Work out the finished part from the listing and answer in its coordinate system (mm). Face numbers are marked on the shaded views. Give positions to 0.01 mm unless a question says otherwise; leave off trailing zeros. Write each loop counter-clockwise with the first axis right and the second up, starting at its lowest first coordinate (ties: lowest second). Pieces come first, ordered by that corner, then holes. Notation, with made-up numbers: (7, -32) -> (25, -32) arc R25 cw to (25, -10) -> close; hole circle Ø8 at (-21.75, 58). An arc over 180 degrees is marked (long way). Use a Markdown table: item, result. Add a question column.
Q1. For a pull along X with two mould halves and no side action, classify the marked faces 1 and 2 as pulls with the +X half, pulls with the -X half, needs draft (parallel to the pull), parting line crosses it, or undercut.
Q2. Section B-B, the plane x = -1 is taken. Give the vertices of the cut face in (y, z) (3 decimals), plus the area to 3 significant figures.
Q3. Section D-D, the plane z = 0.85 is taken. Give the vertices of the cut face in (x, y), plus the area to 3 significant figures.
Q4. Section A-A, the plane y = -2.15 is taken. Give the vertices of the cut face in (x, z) (3 decimals), plus the area to 3 significant figures.
Q5. Consider line 1 (X direction, y = 2.35, z = 0.1) (3 decimals); line 2 (Z direction, x = 2.75, y = 0); line 3 (Y direction, x = 2.25, z = 0.15). Determine where each line is inside the solid, lowest interval first.
Q6. Section C-C, the plane z = 0.4 is taken. Give the vertices of the cut face in (x, y).
from build123d import *

# Parameters (mm, degrees)
SKETCH001_W     = 5.89
SKETCH001_H     = 4.9
PAD001_DEPTH    = 1.04
POCKET_DEPTH    = 6
POCKET001_DEPTH = 6
SKETCH_W        = 0.61
SKETCH_H        = 0.41
PAD_DEPTH       = 0.05
CHAMFER004_SIZE = 0.2
CHAMFER005_SIZE = 0.2
CHAMFER006_SIZE = 0.2
CHAMFER007_SIZE = 0.2


with BuildPart() as pocket001:
    # Sketch001 → Pad001 (new body)
    with BuildSketch(Plane.XY.offset(0.05)):
        with Locations((3.075, 2.575)):
            Rectangle(SKETCH001_W, SKETCH001_H)
    extrude(amount=PAD001_DEPTH)

    # Sketch002 → Pocket (cut)
    with BuildSketch(Plane(origin=(0, 0.125, 0.05), x_dir=(1, 0, 0), z_dir=(0, -1, 0))):
        Polygon((0.13, 0.28), (0.13, 1.04), (0.291543, 1.04), align=None)
        Polygon((5.858457, 1.04), (6.02, 1.04), (6.02, 0.28), align=None)
    extrude(amount=-POCKET_DEPTH, mode=Mode.SUBTRACT)

    # Sketch003 → Pocket001 (cut)
    with BuildSketch(Plane(origin=(6.02, 0, 0.05), x_dir=(0, 1, 0), z_dir=(1, 0, 0))):
        Polygon((0.125, 0.28), (0.125, 1.04), (0.286543, 1.04), align=None)
        Polygon((4.863457, 1.04), (5.025, 1.04), (5.025, 0.28), align=None)
    extrude(amount=-POCKET001_DEPTH, mode=Mode.SUBTRACT)


with BuildPart() as fusion:
    # Sketch → Pad (new body)
    with BuildSketch(Plane.XY):
        Polygon((3.52, 0), (3.52, 0.49), (0, 0.49), (0, 0.9), (0.61, 0.9), (0.61, 1.743333), (0, 1.743333), (0, 2.153333), (0.61, 2.153333), (0.61, 2.996667), (0, 2.996667), (0, 3.406667), (0.61, 3.406667), (0.61, 4.25), (0, 4.25), (0, 4.66), (3.52, 4.66), (3.52, 5.15), (4.27, 5.15), (4.27, 0), align=None)
        with Locations((5.845, 4.455)):
            Rectangle(SKETCH_W, SKETCH_H)
        with Locations((5.845, 3.201667)):
            Rectangle(SKETCH_W, SKETCH_H)
        with Locations((5.845, 1.948333)):
            Rectangle(SKETCH_W, SKETCH_H)
        with Locations((5.845, 0.695)):
            Rectangle(SKETCH_W, SKETCH_H)
    extrude(amount=PAD_DEPTH)

    # Chamfer004
    chamfer004_edges = [fusion.edges().sort_by_distance(p)[0] for p in [
        (4.27, 0, 0.025),
    ]]
    chamfer(chamfer004_edges, length=CHAMFER004_SIZE)

    # Chamfer005
    chamfer005_edges = [fusion.edges().sort_by_distance(p)[0] for p in [
        (3.52, 0, 0.025),
    ]]
    chamfer(chamfer005_edges, length=CHAMFER005_SIZE)

    # Chamfer006
    chamfer006_edges = [fusion.edges().sort_by_distance(p)[0] for p in [
        (3.52, 5.15, 0.025),
    ]]
    chamfer(chamfer006_edges, length=CHAMFER006_SIZE)

    # Chamfer007
    chamfer007_edges = [fusion.edges().sort_by_distance(p)[0] for p in [
        (4.27, 5.15, 0.025),
    ]]
    chamfer(chamfer007_edges, length=CHAMFER007_SIZE)

    # Fusion: union Pocket001
    add(pocket001.part)


with BuildPart() as fusion_1:
    # Fusion placement: moved
    add(fusion.part.moved(Location((-3.075, -2.575, 0))))


solid = fusion_1.part
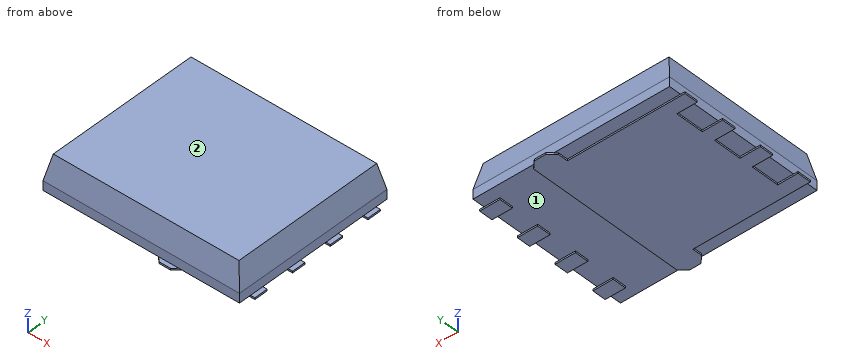
Result set:
| question | item | result |
|---|---|---|
| 1 | face 1 | undercut |
| 1 | face 2 | needs draft |
| 2 | outline | (-2.45, 0.05) -> (-2.085, 0.05) -> (-2.085, 0) -> (2.085, 0) -> (2.085, 0.05) -> (2.45, 0.05) -> (2.45, 0.33) -> (2.288, 1.09) -> (-2.288, 1.09) -> (-2.45, 0.33) -> close |
| 2 | area | 5.18 mm2 |
| 3 | outline | (-2.83, -2.34) -> (2.83, -2.34) -> (2.83, 2.34) -> (-2.83, 2.34) -> close |
| 3 | area | 26.5 mm2 |
| 4 | outline | (-2.945, 0.05) -> (0.445, 0.05) -> (0.445, 0) -> (1.195, 0) -> (1.195, 0.05) -> (2.945, 0.05) -> (2.945, 0.33) -> (2.783, 1.09) -> (-2.783, 1.09) -> (-2.945, 0.33) -> close |
| 4 | area | 6.04 mm2 |
| 5 | line 1 | x = -2.945 to 2.945 |
| 5 | line 2 | z = 0.05 to 1.09 |
| 5 | line 3 | y = -2.45 to 2.45 |
| 6 | outline | (-2.93, -2.44) -> (2.93, -2.44) -> (2.93, 2.44) -> (-2.93, 2.44) -> close |
